Input: part model. Units: mm. Frame: model coordinates. A direction names the side the tool comes from. Round coordinates to 2 decimals unless told otherwise and drop trailing zeros. Loops run counter-clockwise (first coordinate to the right, second up) from the corner with the lowest first, then second, coordinate; pieces in that order, holes last.
1) Access query for faces 4 (the face through (0, 15, 384)), 5 (the face through (-17.5, 0, 384)). Directions: +Z, -Z, +X, -X, +Y, -Y. A direction counts if a zero-diameter tool reaches every point of the face in a straight line with its end or side. Return the directions, or none.
2) First-contact query: pin 1 (13 mm diameter, centred on y = 0, z = 687.5, fed in from +X). Flat tip, straight axial feed; report the tip coordinate or a pass-through.
3) Draft query along Y for faces 1 (the face through (0, -15, 385)), 2 (the face through (0, 17.5, 384)), 3 (the face through (17.5, 0, 384)). Return one class per face: pulls with the +Y half, pulls with the -Y half, needs draft (parallel to the pull), parting line crosses it, or undercut.
4) Section A-A, the plane x = -1.5. Return loops of the section in (y, z).
5) Ray query, line 1 along X through (y, z) = (-10, 548.5); line 2 along Z through (x, y) = (16.25, 0). Return the intervals inside material, ascending.
6) Section B-B, the plane z = 435. Return loops of the section in (x, y).
Autodesk Inventor part; units mm, degrees
ref_plane "Start plane" through (0, 0, -17.5) normal (0, 0, 1) x (1, 0, 0)
ref_plane "End plane" through (0, 0, 797.5) normal (0, 0, 1) x (1, 0, 0)
ref_plane "Work Plane4" through (-17.5, 0, -17.5) normal (0, 0, -1) x (-1, 0, 0)
ref_plane "Start plane" through (0, 0, -17.5) normal (0, 0, 1) x (1, 0, 0)
ref_plane "End plane" through (0, 0, 797.5) normal (0, 0, 1) x (1, 0, 0)
sketch "Sketch" plane through (0, 0, 0) normal (0, 0, 1) x (1, 0, 0)
  line L0 (-17.5, -12.5) -> (-17.5, 12.5)
  line L1 (-12.5, 17.5) -> (12.5, 17.5)
  line L2 (17.5, 12.5) -> (17.5, -12.5)
  line L3 (12.5, -17.5) -> (-12.5, -17.5)
  arc A0 (-17.5, -12.5) -> (-12.5, -17.5) centre (-12.5, -12.5) ccw
  arc A1 (-12.5, 17.5) -> (-17.5, 12.5) centre (-12.5, 12.5) ccw
  arc A2 (17.5, 12.5) -> (12.5, 17.5) centre (12.5, 12.5) ccw
  arc A3 (12.5, -17.5) -> (17.5, -12.5) centre (12.5, -12.5) ccw
  arc A4 (-12.5, 15) -> (-15, 12.5) centre (-12.5, 12.5) ccw
  line L4 (-12.5, 15) -> (12.5, 15)
  arc A5 (15, 12.5) -> (12.5, 15) centre (12.5, 12.5) ccw
  line L5 (15, 12.5) -> (15, -12.5)
  arc A6 (12.5, -15) -> (15, -12.5) centre (12.5, -12.5) ccw
  line L6 (12.5, -15) -> (-12.5, -15)
  arc A7 (-15, -12.5) -> (-12.5, -15) centre (-12.5, -12.5) ccw
  line L7 (-15, -12.5) -> (-15, 12.5)
  line L8 (0, 25.9497) -> (0, -25.9497) construction
  line L9 (-25.9497, 0) -> (25.9497, 0) construction
  dimension "d7" = 5
  dimension "d10" = 35
  dimension "d11" = 35
  dimension "d12" = 2.5
  dimension "d15" = 17.5
  dimension "d16" = 17.5
extrude "Body" add sketch "Sketch" along normal up to surface (815 mm away) from surface at -17.5
sketch "Sketch3" plane through (0, 0, 0) normal (0, 0, 1) x (1, 0, 0)
  line L0 (0, 0) -> (10, 0)
ref_plane "Work Plane3" through (0, 0, 0) normal (0, -1, 0) x (1, 0, 0)
sketch "Sketch4" plane through (0, 0, 0) normal (0, -1, 0) x (1, 0, 0)
  line L0 (-2, -17.5) -> (12, -17.5)
  line L1 (-2, 797.5) -> (12, 797.5)
  dimension "d18" = 815
ref_plane "Work Plane4" through (-17.5, 0, -17.5) normal (0, 0, -1) x (-1, 0, 0)
split "Split1" plane through (-17.5, 0, -17.5) removes the side toward (0, 0, -1)
ref_plane "Work Plane5" through (-107.5, 0, 797.5) normal (0, 0, 1) x (1, 0, 0)
split "Split2" plane through (-107.5, 0, 797.5) removes the side toward (0, 0, 1)
ref_plane "Work Plane6" through (0, 17.5, -17.5) normal (0, -0.7071, -0.7071) x (1, 0, 0)
split "Split3" plane through (0, 17.5, -17.5) removes the side toward (0, -0.7071, -0.7071)
ref_plane "Work Plane8" through (0, 17.5, 797.5) normal (0, -0.7071, 0.7071) x (1, 0, 0)
split "Split5" plane through (0, 17.5, 797.5) removes the side toward (0, -0.7071, 0.7071)
sketch "Sketch5" plane through (17.5, 12.5, 792.5) normal (1, 0, 0) x (0, 0, -1)
  line L0 (0, 0) -> (25, -25) construction
  line L1 (25, -25) -> (780, -25) construction
  line L2 (780, -25) -> (805, 0) construction
  line L3 (0, 0) -> (805, 0) construction
  line L4 (30, -475) -> (30, -30) construction
  line L5 (775, -30) -> (775, -95) construction
  line L6 (105, 0) -> (105, -25) construction
  line L7 (25, -25) -> (780, -25) construction
  line L8 (216.5, 0) -> (216.5, -25) construction
  line L9 (105, -12.5) -> (216.5, -12.5) construction
  line L10 (700, 0) -> (700, -25) construction
  line L11 (0, 0) -> (805, 0) construction
  line L12 (588.5, 0) -> (588.5, -25) construction
  line L13 (588.5, -12.5) -> (700, -12.5) construction
  point P0 (792.5, -12.5)
  point P1 (15, 0)
  dimension "d19" = 75
  dimension "d20" = 111.5
  dimension "d21" = 75
  dimension "d22" = 111.5
hole "Hole1" at (17.5, 0, 687.5) at (17.5, 0, 576) at (17.5, 0, 204) at (17.5, 0, 92.5) direction (-1, 0, 0) diameter 10 end through all
equation "\"d7\" = G_IR"
equation "\"d10\" = G_H"
equation "\"d11\" = G_W"
equation "\"d12\" = G_T"
equation "\"d15\" = 0.5 * d10"
equation "\"d16\" = 0.5 * d11"
equation "\"d3\" = G_L"
equation "\"G_W\" = 35"
equation "\"G_H\" = 35"
equation "\"G_T\" = 2.5"
equation "\"G_IR\" = 5"
equation "\"G_L\" = d18"
equation "\"G_OFFSET_START\" = 17.5"
equation "\"G_OFFSET_END\" = 17.5"
equation "\"d13\" = -G_OFFSET_START"
equation "\"d14\" = G_OFFSET_END + B_L"
properties part number "AS 1163 - C350L0 35x35x2.5 SHS - 815" material "Steel, Mild"
Final values:
1. face 4: +Z, -Z
1. face 5: +Z, -Z, -X, +Y, -Y
2. pin 1: stops at x = 17.5
3. face 1: undercut
3. face 2: pulls with the +Y half
3. face 3: needs draft
4. outline: (-17.5, 17.5) - (-15, 15) - (-15, 765) - (-17.5, 762.5) - close; (15, -15) - (17.5, -17.5) - (17.5, 797.5) - (15, 795) - close
5. line 1: x = -17.5 to -15, 15 to 17.5
5. line 2: z = 0 to 87.5, 97.5 to 199, 209 to 571, 581 to 682.5, 692.5 to 780
6. outline: (-17.5, -12.5) arc R5 ccw to (-12.5, -17.5) - (12.5, -17.5) arc R5 ccw to (17.5, -12.5) - (17.5, 12.5) arc R5 ccw to (12.5, 17.5) - (-12.5, 17.5) arc R5 ccw to (-17.5, 12.5) - close; hole (-15, -12.5) arc R2.5 ccw to (-12.5, -15) - (12.5, -15) arc R2.5 ccw to (15, -12.5) - (15, 12.5) arc R2.5 ccw to (12.5, 15) - (-12.5, 15) arc R2.5 ccw to (-15, 12.5) - close
